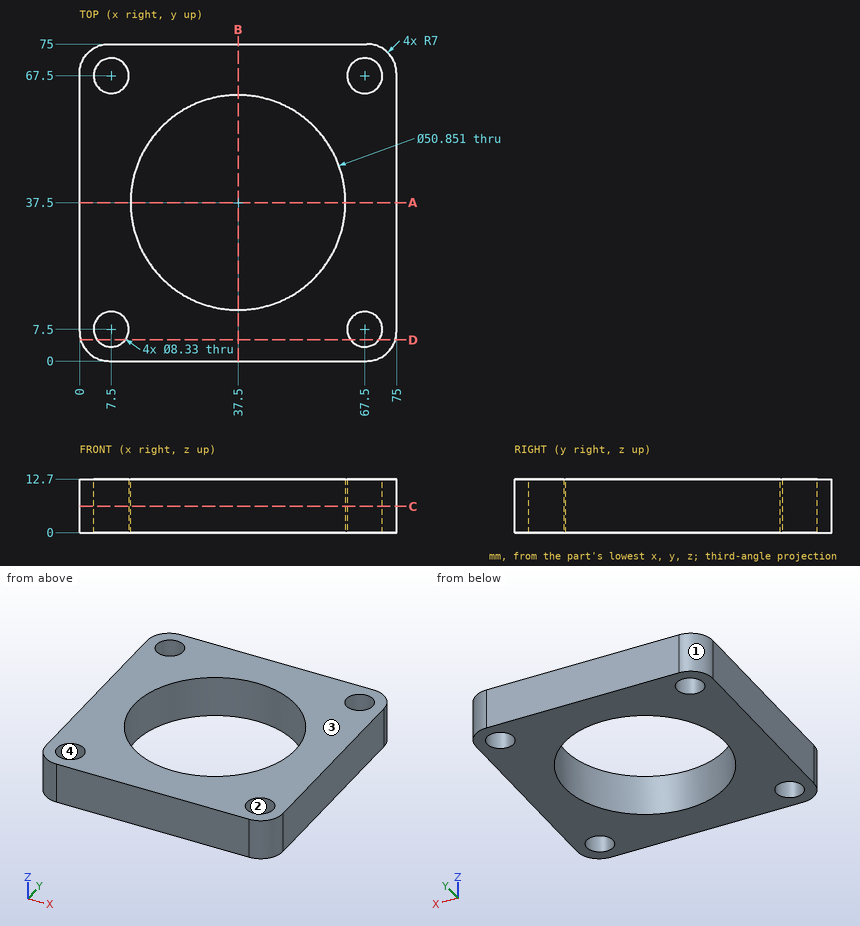
Job drawing, mm, ordinate dimensions from the low corner. One solid piece. Coordinates: 2 decimals unless noted, no trailing zeros. Order: outer loops, then holes, each group sorted by start corner. A loop starts at its lowest first (then second) coordinate and runs counter-clockwise, first axis right, second up. Notation, with made-up numbers: (27.25, 87) - (53.25, 87) arc R27 cw to (53.25, 117) - close; hole circle Ø3 at (46.25, 77.5). An arc over 180 degrees is marked (long way). Return JSON: item names as keys, results as strings. Group by question number.
1) Saw through at D-D, the plane y = 5. Write the cut outline in (x, z), plus the area to 3 significant figures.
2) Mould opens along X. For the marked faces 1, 2, 3 and 4 say: released by +X, released by -X, zero draft, split by the parting line, or undercut.
3) Saw through at C-C, the plane z = 6.25. Write the cut outline in (x, y) (1 decimal), plus the area to 3 significant figures.
4) Saw through at A-A, the plane y = 37.5. Write the cut outline in (x, z) (1 decimal), plus the area to 3 significant figures.
5) Probe line 1 (X direction, y = 7.5, z = 3.25) (3 decimals); line 2 (Y direction, x = 37.5, z = 6.75) (1 decimal). List the from-to ranges inside material, lowest first. Write a range as from..to.
Values found:
{
 "1": {"outline": "(0.29, 0) - (4.17, 0) - (4.17, 12.7) - (0.29, 12.7) - close; (10.83, 0) - (64.17, 0) - (64.17, 12.7) - (10.83, 12.7) - close; (70.83, 0) - (74.71, 0) - (74.71, 12.7) - (70.83, 12.7) - close", "area": "776 mm²"},
 "2": {"face 1": "released by -X", "face 2": "undercut", "face 3": "zero draft", "face 4": "undercut"},
 "3": {"outline": "(0, 7) arc R7 ccw to (7, 0) - (68, 0) arc R7 ccw to (75, 7) - (75, 68) arc R7 ccw to (68, 75) - (7, 75) arc R7 ccw to (0, 68) - close; hole circle Ø8.3 at (7.5, 7.5); hole circle Ø8.3 at (7.5, 67.5); hole circle Ø50.9 at (37.5, 37.5); hole circle Ø8.3 at (67.5, 7.5); hole circle Ø8.3 at (67.5, 67.5)", "area": "3,330 mm²"},
 "4": {"outline": "(0, 0) - (12.1, 0) - (12.1, 12.7) - (0, 12.7) - close; (62.9, 0) - (75, 0) - (75, 12.7) - (62.9, 12.7) - close", "area": "307 mm²"},
 "5": {"line 1": "x = 0..3.335, 11.665..63.335, 71.665..75", "line 2": "y = 0..12.1, 62.9..75"}
}
